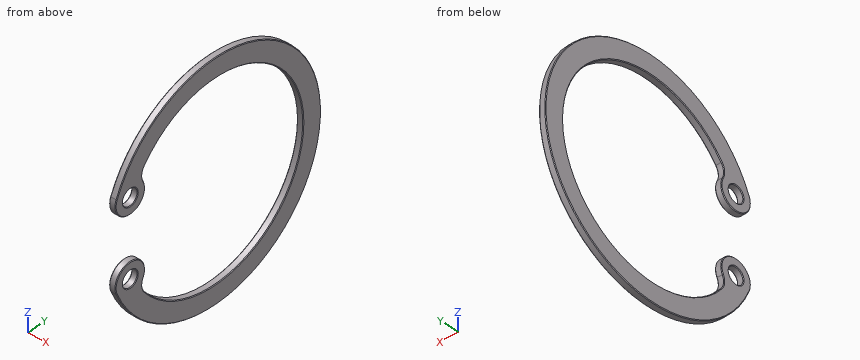
Autodesk Inventor part; units mm, degrees
ref_plane "YZ Plane" through (0, 0, 0) normal (1, 0, 0) x (0, 1, 0)
ref_plane "XZ Plane" through (0, 0, 0) normal (0, 1, 0) x (-1, 0, 0)
ref_plane "XY Plane" through (0, 0, 0) normal (0, 0, 1) x (1, 0, 0)
sketch "Szkic1" plane through (0, 0, 0) normal (1, 0, 0) x (0, 1, 0)
  arc A0 (-8.3149, -3.4442) -> (-8.3149, 3.4442) centre (0, 0) ccw
  arc A1 (-6.9291, -2.8701) -> (-6.694, -3.3823) centre (0, 0) ccw construction
  line L0 (0, 0) -> (-6.5826, 2.7266)
  line L1 (0, 0) -> (-6.5826, -2.7266)
  line L2 (-11.9129, 0) -> (12.4855, 0)
  circle A2 centre (-7.1601, 2.9658) radius 0.625
  line L3 (-6.9291, 2.8701) -> (-7.1601, 2.9658) construction
  arc A3 (-8.3149, 3.4442) -> (-6.0415, 3.5238) centre (-7.1601, 2.9658) ccw
  circle A4 centre (-7.1601, -2.9658) radius 0.625
  arc A5 (-6.3801, -3.9426) -> (-6.0415, -3.5238) centre (-7.1601, -2.9658) ccw construction
  arc A6 (-6.694, -3.3823) -> (-6.3801, -3.9426) centre (0, 0) ccw construction
  arc A7 (-6.3801, -3.9426) -> (-5.9385, -4.5809) centre (0, 0) ccw construction
  arc A8 (-6.694, 3.3823) -> (-6.9291, 2.8701) centre (0, 0) ccw construction
  line L4 (-6.5826, 2.7266) -> (-8.3149, 3.4442) construction
  line L5 (-6.5826, -2.7266) -> (-8.3149, -3.4442) construction
  arc A9 (-6.3801, 3.9426) -> (-6.694, 3.3823) centre (0, 0) ccw construction
  arc A10 (-5.9385, 4.5809) -> (-6.0415, 3.5238) centre (-5.1467, 3.9701) ccw
  arc A11 (-6.0415, -3.5238) -> (-5.9385, -4.5809) centre (-5.1467, -3.9701) ccw
  arc A12 (-5.9385, 4.5809) -> (-6.3801, 3.9426) centre (0, 0) ccw construction
  arc A13 (-6.0415, 3.5238) -> (-6.3801, 3.9426) centre (-7.1601, 2.9658) ccw construction
  arc A14 (-6.0415, -3.5238) -> (-8.3149, -3.4442) centre (-7.1601, -2.9658) ccw
  arc A15 (-5.9385, -4.5809) -> (-5.9385, 4.5809) centre (0, 0) ccw
  dimension "d0" = 18
  dimension "d1" = 15
  dimension "d2" = 45
  dimension "d3" = 1.25
  dimension "d4" = 0.25
  dimension "d5" = 2
extrude "Wyciągnięcie proste1" add sketch "Szkic1" along normal blind 0.5 contours A14 A11 A15 L2 A0 | L2 A15 A10 A3 A0
chamfer "Faza1" distance 0.05 angle 45 16 edges at (0.5, 7.5, 0) (0.5, -6.1419, -4.0672) (0.5, -7.1163, -1.7166) (0.5, 9, 0) (0.5, -7.1163, 1.7166) (0.5, -6.1419, 4.0672) (0, 7.5, 0) (0, -6.1419, -4.0672) (0, -7.1163, -1.7166) (0, 9, 0) (0, -7.1163, 1.7166) (0, -6.1419, 4.0672) (0, -7.7851, 2.9658) (0.5, -7.7851, 2.9658) (0, -7.7851, -2.9658) (0.5, -7.7851, -2.9658)
properties part number "Seger"
Input: part model. Units: mm. Frame: model coordinates. Coordinates: 2 decimals unless noted, no trailing zeros. Write each loop counter-clockwise with the first axis right and the second up, starting at its lowest first coordinate (ties: lowest second). Pieces come first, ordered by that corner, then holes.
1) Material intervals for line 1 along Z through (x, y) = (0.2, 0); line 2 along Y through (x, z) = (0.2, 2.5); line 3 along Y through (x, z) = (0.35, 3.25), sorted ascending.
2) Section A-A on y = 0. Output: boundary loops of the cut face in (x, z), and give its area (3 significant figures).
3) Section B-B on z = 0. Output: boundary loops of the cut face in (x, y), and give its area (3 significant figures).
4) Section C-C on x = 0.3. State how many separate pieces and enclosed holes the cut face has, and give its area (3 significant figures).
Check result:
1. line 1: z = -9 to -7.5, 7.5 to 9
1. line 2: y = -8.32 to -7.58, -6.74 to -6, 7.07 to 8.65
1. line 3: y = -8.38 to -7.72, -6.6 to -5.94, 6.76 to 8.39
2. outline: (0, -8.95) - (0.05, -9) - (0.45, -9) - (0.5, -8.95) - (0.5, -7.55) - (0.45, -7.5) - (0.05, -7.5) - (0, -7.55) - close; (0, 7.55) - (0.05, 7.5) - (0.45, 7.5) - (0.5, 7.55) - (0.5, 8.95) - (0.45, 9) - (0.05, 9) - (0, 8.95) - close
2. area: 1.49 mm2
3. outline: (0, 7.55) - (0.05, 7.5) - (0.45, 7.5) - (0.5, 7.55) - (0.5, 8.95) - (0.45, 9) - (0.05, 9) - (0, 8.95) - close
3. area: 0.745 mm2
4. separate pieces: 1
4. enclosed holes: 2
4. area: 72.4 mm2
